from build123d import *

# Parameters (mm, degrees)
SKETCH_1_R          = 20
SKETCH_1_R_2        = 4
EXTRUDE_1_DEPTH     = 25
SKETCH_2_R          = 12
CUT_EXTRUDE_1_DEPTH = 8
CUT_EXTRUDE_START   = -8
SKETCH_3_R          = 12
CUT_EXTRUDE_2_DEPTH = 8


with BuildPart() as part:
    # 草图1 → 凸台-拉伸1 (new body)
    with BuildSketch(Plane.XY):
        with Locations((-43.920622876, 23.400003441)):
            Circle(SKETCH_1_R)
        with Locations((-43.920622876, 23.400003441)):
            Circle(SKETCH_1_R_2, mode=Mode.SUBTRACT)
    extrude(amount=EXTRUDE_1_DEPTH)

    # 草图2 → 切除-拉伸1 (cut)
    with BuildSketch(Plane.XY.offset(25)):
        with Locations((-43.920622876, 23.400003441)):
            Circle(SKETCH_2_R)
    extrude(amount=-CUT_EXTRUDE_1_DEPTH, mode=Mode.SUBTRACT)

    # 草图3 → 切除-拉伸2 (cut)
    with BuildSketch(Plane(origin=(0, 0, 0), x_dir=(-1, 0, 0), z_dir=(0, 0, -1)).offset(CUT_EXTRUDE_START)):
        with Locations(Location((43.920622876, 23.400003441, 0), (0, 0, 180))):
            Circle(SKETCH_3_R)
    extrude(amount=CUT_EXTRUDE_2_DEPTH, mode=Mode.SUBTRACT)


solid = part.part
Can you work these out from the model? Positions are in its coordinate system, mm. A direction names the side the tool comes from. Give positions to 0.01 mm unless a question says otherwise; leave off trailing zeros. Order: outer loops, then holes, each group sorted by start corner. A loop starts at its lowest first (then second) coordinate and runs counter-clockwise, first axis right, second up. Notation, with made-up numbers: M 8.25,40 L 43.25,40 A16 ccw 43.25,61 Z; hole C 70.25,-21 d9. An arc over 180 degrees is marked long. Use one line per item in the form item = value.
Item 1: If we section it at A-A, the plane z = 11.25: Write out the boundary of the cut face in (x, y).
Values follow:
outline = C -43.92,23.4 d40; hole C -43.92,23.4 d8
Item 2: If I drill on line 1 along Z through (x, y) = (-34, 25); line 2 along X through (y, z) = (34.5, 6.25); line 3 along Y through (x, z) = (-52.5, 18.25), over which ranges is the centre line in solid material (lowest first)? Write a range as [from, to].
Values follow:
line_1 = [8, 17]
line_2 = [-60.56, -48.48], [-39.36, -27.28]
line_3 = [5.33, 15.01], [31.79, 41.47]
Item 3: If we section it at C-C, the plane y = 22: Write out the boundary of the cut face in (x, z).
Values follow:
outline = M -63.87,0 L -55.84,0 L -55.84,8 L -47.67,8 L -47.67,17 L -55.84,17 L -55.84,25 L -63.87,25 Z; M -40.17,8 L -32,8 L -32,0 L -23.97,0 L -23.97,25 L -32,25 L -32,17 L -40.17,17 Z
Item 4: Will these pins go through, and if not, where does the flat tip stop? pin 1 Ø19 at (x, y) = (-43.92, 23.4) entering from -Z; pin 2 Ø5 at (x, z) = (-57.5, 22.5) entering from -Y; pin 3 Ø2 at (x, z) = (-43.5, 19) entering from +Y.
Values follow:
pin_1 = 8
pin_2 = 6.75
pin_3 = 43.4
Item 5: Thinking about a two-plate mould opening in Y: for faces 1 (the cylindrical face through (-25.446, 15.74, 12.325)), 2 (the flat face through (-35, 15, 25)), 3 (the cylindrical face through (-52.765, 15.29, 4.056)), which applies, pulls with the +Y half, pulls with the -Y half, needs draft (parallel to the pull), parting line crosses it, or undercut?
Values follow:
face_1 = parting line crosses it
face_2 = needs draft
face_3 = undercut
Item 6: If we section it at D-D, the plane y = 18: Write out the boundary of the cut face in (x, z).
Values follow:
outline = M -63.18,0 L -54.64,0 L -54.64,8 L -33.2,8 L -33.2,0 L -24.66,0 L -24.66,25 L -33.2,25 L -33.2,17 L -54.64,17 L -54.64,25 L -63.18,25 Z
Item 7: For faces 4 (the flat face through (-44, 29, 8)), 5 (the cylindrical face through (-40.226, 21.868, 12.437)), 6 (the flat face through (-39, 24, 17)), which set-ups out of +Z, -Z, +X, -X, +Y, -Y let a thin tool reach every point of the face, with its end or its side?
Values follow:
face_4 = -Z
face_5 = +Z, -Z
face_6 = +Z
Item 8: If we section it at B-B, the plane x = -43: Write out the boundary of the cut face in (y, z), and give its area (3 significant figures).
Values follow:
outline = M 3.42,0 L 11.44,0 L 11.44,8 L 19.51,8 L 19.51,17 L 11.44,17 L 11.44,25 L 3.42,25 Z; M 27.29,8 L 35.36,8 L 35.36,0 L 43.38,0 L 43.38,25 L 35.36,25 L 35.36,17 L 27.29,17 Z
area = 546 mm^2
